from build123d import *

# Parameters (mm, degrees)
F0_W     = 101.6
F0_H     = 12.7
F1_DEPTH = 228.6
F2_R     = 5
F3_DEPTH = 12.701


with BuildPart() as f1:
    # F0 (on Front) → F1 (new body)
    with BuildSketch(Plane.XZ):
        with Locations((-9.152951, -4.734359)):
            Rectangle(F0_W, F0_H)
    extrude(amount=F1_DEPTH)

    # F2 (on face) → F3 (cut, through all)
    with BuildSketch(Plane.XY.offset(1.615641)):
        with Locations((34.361049, -56.4097)):
            Circle(F2_R)
        with Locations((34.361049, -172.1905)):
            Circle(F2_R)
        with Locations((-37.640351, -56.4097)):
            Circle(F2_R)
        with Locations((-37.640351, -172.1905)):
            Circle(F2_R)
        with Locations((-37.953511, -212.725)):
            Circle(F2_R)
        with Locations((-37.953511, -15.875)):
            Circle(F2_R)
    extrude(amount=-F3_DEPTH, mode=Mode.SUBTRACT)


solid = f1.part
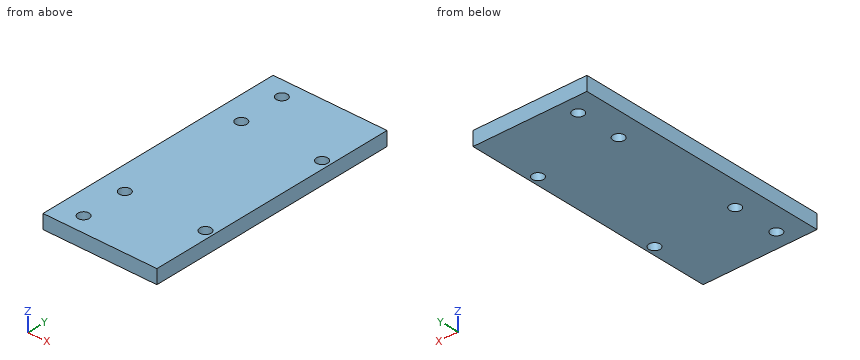
Can you work these out from the model? Positions are in its coordinate system, mm. Coordinates: 2 decimals unless noted, no trailing zeros. Write each loop counter-clockwise with the first axis right and the second up, starting at its lowest first coordinate (ties: lowest second). Pieces come first, ordered by that corner, then holes. Notation, with made-up numbers: (70.5, 26.5) -> (116.5, 26.5) arc R19 cw to (116.5, 38.5) -> close; hole circle Ø3 at (-25.5, 8). An arc over 180 degrees is marked (long way). Write each question's results on one line, items separated by ' | '. Start each with the question number.
Q1. I'm going to push a flat-ended pin straight in: pin 1 (13 mm diameter, centred on x = -37.64, y = -172.19, fed in from -Z). Where does the tip first touch, or does it pass through?
Q2. Imagine slicing it at B-B (z = -8.25). Write out the boundary of the cut face in (x, y) (1 decimal), then the cut area to 3 significant figures.
Q3. Imagine slicing it at A-A (x = -35). Write out the boundary of the cut face in (y, z), then the cut area to 3 significant figures.
Q4. If I drill on probe 1 along Y at (x, z) = (35, -7.25); probe 2 along X at (y, z) = (-175.5, -7); probe 3 along X at (y, z) = (-212.5, -6.25), over which ranges is the centre line in solid material (lowest first)?
Taken from the geometry:
1) pin 1: stops at z = -11.08
2) outline: (-60, -228.6) -> (41.6, -228.6) -> (41.6, 0) -> (-60, 0) -> close; hole circle Ø10 at (-38, -212.7); hole circle Ø10 at (-38, -15.9); hole circle Ø10 at (-37.6, -172.2); hole circle Ø10 at (-37.6, -56.4); hole circle Ø10 at (34.4, -172.2); hole circle Ø10 at (34.4, -56.4) | area: 22,800 mm^2
3) outline: (-228.6, -11.08) -> (-216.76, -11.08) -> (-216.76, 1.62) -> (-228.6, 1.62) -> close; (-208.69, -11.08) -> (-176.44, -11.08) -> (-176.44, 1.62) -> (-208.69, 1.62) -> close; (-167.94, -11.08) -> (-60.66, -11.08) -> (-60.66, 1.62) -> (-167.94, 1.62) -> close; (-52.16, -11.08) -> (-19.91, -11.08) -> (-19.91, 1.62) -> (-52.16, 1.62) -> close; (-11.84, -11.08) -> (0, -11.08) -> (0, 1.62) -> (-11.84, 1.62) -> close | area: 2,480 mm^2
4) probe 1: y = -228.6 to -177.15, -167.23 to -61.37, -51.45 to 0 | probe 2: x = -59.95 to -41.39, -33.89 to 30.61, 38.11 to 41.65 | probe 3: x = -59.95 to -42.95, -32.96 to 41.65
